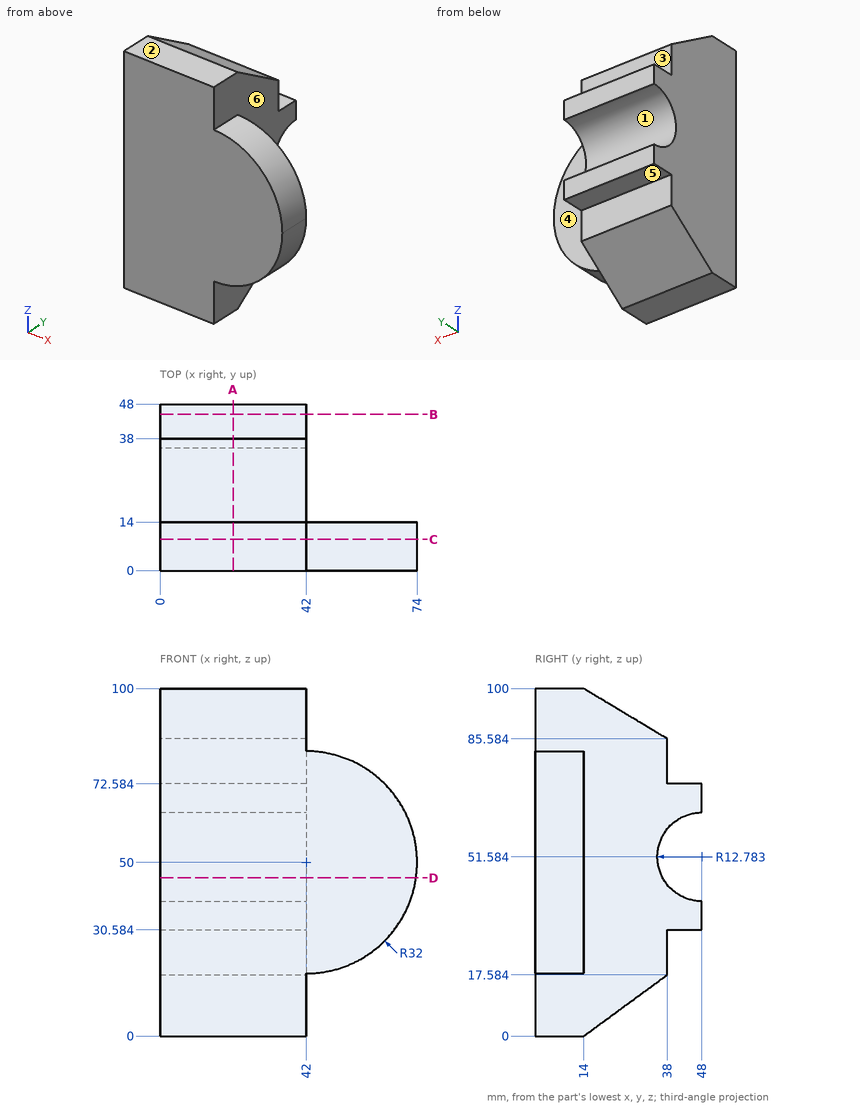
Geometry: see drawing. Coordinates: mm, zero at the bounding-box minimum. A direction names the side the tool comes from. Give positions to 0.01 mm unless a question says otherwise; leave off trailing zeros. Loops run counter-clockwise (first coordinate to the right, second up) from the corner with the lowest first, then second, coordinate; pieces in that order, holes last. Notation, with made-up numbers: (-34, 4) - (-7, 4) arc R22 cw to (-7, 43) - close; hole circle Ø7 at (-23.75, -20). An arc over 180 degrees is marked (long way). One line per question, with ' | ' between items. Start each with the question number.
(1) Section query A-A on x = 21. Return loops of the section in (y, z).
(2) Pull-direction query (Z, two-part tool) for the marked faces 1, 2 and 3; classes: released by +Z, released by -Z, zero draft, split by the parting line, or undercut.
(3) Section query D-D on z = 45.5. Return loops of the section in (x, y), then the cut area to 3 significant figures.
(4) Reachability of the marked faces 4, 5 and 6 from +Z, -Z, +X, -X, +Y, -Y: full face, straight path, thin tool, end or side. Return the list, or none.
(5) Section query C-C on y = 9. Return loops of the section in (x, z), then the cut area to 3 significant figures.
(6) Ray query, line 1 (X direction, y = 37.5, z = 29); line 2 (Y direction, x = 13.5, z = 77.5); line 3 (Y direction, x = 58.5, z = 76.5). Return the intervals inside material, ascending. Write a range as from..to.
(7) Contact query for flat-ended pins moving along their axis: pin 1 (8 mm diameter, centred on x = 19.5, y = 40.5, fed in from -Z) (3 decimals); pin 2 (1 mm diameter, centred on y = 43, z = 32, fed in from +X); pin 3 (16 mm diameter, centred on x = 65, z = 58.5, fed in from +Y); pin 4 (12 mm diameter, centred on x = 58.5, z = 12, fed in from -Y). Output: stop coordinate, or through.
(8) Section query B-B on y = 45. Return loops of the section in (x, z).
The answers:
1) outline: (0, 0) - (14, 0) - (38, 17.58) - (38, 30.58) - (48, 30.58) - (48, 38.8) arc R12.78 cw to (48, 64.37) - (48, 72.58) - (38, 72.58) - (38, 85.58) - (14, 100) - (0, 100) - close
2) face 1: undercut | face 2: released by +Z | face 3: zero draft
3) outline: (0, 0) - (73.68, 0) - (73.68, 14) - (42, 14) - (42, 36.76) - (0, 36.76) - close | area: 1,990 mm2
4) face 4: +Z, -Z, +X, +Y | face 5: -Z, +X, -X, +Y | face 6: +X, +Y
5) outline: (0, 0) - (42, 0) - (42, 18) arc R32 ccw to (42, 82) - (42, 100) - (0, 100) - close | area: 5,810 mm2
6) line 1: 0..42 | line 2: 0..38 | line 3: 0..14
7) pin 1: z = 16.485 | pin 2: x = 42 | pin 3: y = 14 | pin 4: through
8) outline: (0, 30.58) - (42, 30.58) - (42, 39.16) - (0, 39.16) - close; (0, 64.01) - (42, 64.01) - (42, 72.58) - (0, 72.58) - close
